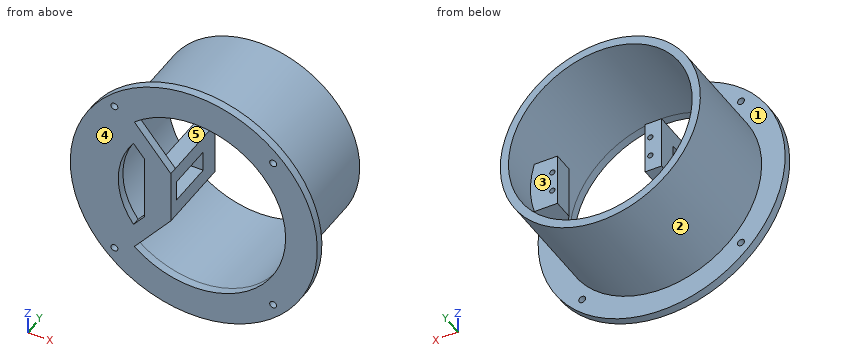
```python
from build123d import *

# Parameters (mm, degrees)
SKETCH1_R           = 60.5
SKETCH1_R_2         = 1.7
BOSS_EXTRUDE1_DEPTH = 4
SKETCH2_R           = 49
SKETCH2_R_2         = 45
BOSS_EXTRUDE2_DEPTH = 53
SKETCH3_W           = 8
SKETCH3_H           = 26
BOSS_EXTRUDE3_DEPTH = 1
SKETCH4_W           = 8
SKETCH4_H           = 8
BOSS_EXTRUDE4_DEPTH = 23
SKETCH5_W           = 8
SKETCH5_H           = 26
BOSS_EXTRUDE5_DEPTH = 10
SKETCH6_R           = 1.3
CUT_EXTRUDE1_DEPTH  = 5
BOSS_EXTRUDE6_START = -10
SKETCH7_R           = 1.3
BOSS_EXTRUDE6_DEPTH = 10
SKETCH12_R          = 1.3
BOSS_EXTRUDE8_DEPTH = 5
RIB4_REACH          = 104.808
SKETCH17_WALL_W     = 226.415050864
SKETCH17_WALL_H     = 26
SKETCH18_R          = 5
CUT_EXTRUDE3_DEPTH  = 21


with BuildPart() as part:
    # Sketch1 → Boss-Extrude1 (new body)
    with BuildSketch(Plane(origin=(0, 0, 0), x_dir=(-1, 0, 0), z_dir=(0, 1, 0))):
        with Locations(Location((0, 0, 0), (0, 0, 90))):
            Circle(SKETCH1_R)
        with Locations(Location((38.890872965, 38.890872965, 0), (0, 0, 90))):
            Circle(SKETCH1_R_2, mode=Mode.SUBTRACT)
        with Locations(Location((38.890872965, -38.890872965, 0), (0, 0, 90))):
            Circle(SKETCH1_R_2, mode=Mode.SUBTRACT)
        with Locations(Location((-38.890872965, -38.890872965, 0), (0, 0, 90))):
            Circle(SKETCH1_R_2, mode=Mode.SUBTRACT)
        with Locations(Location((-38.890872965, 38.890872965, 0), (0, 0, 90))):
            Circle(SKETCH1_R_2, mode=Mode.SUBTRACT)
        with BuildLine():
            Line((11.25, -13), (11.25, 13))
            Line((11.25, 13), (29.125473669, 34.303159964))
            ThreePointArc((29.125473669, 34.303159964), (-45, 0), (29.125473669, -34.303159964))
            Line((29.125473669, -34.303159964), (11.25, -13))
        make_face(mode=Mode.SUBTRACT)
        with BuildLine():
            Line((24.25, -16), (24.25, 16))
            Line((24.25, 16), (29.530226152, 22.292728487))
            ThreePointArc((29.530226152, 22.292728487), (37, 0), (29.530226152, -22.292728487))
            Line((29.530226152, -22.292728487), (24.25, -16))
        make_face(mode=Mode.SUBTRACT)
    extrude(amount=BOSS_EXTRUDE1_DEPTH)

    # Sketch2 → Boss-Extrude2 (add)
    with BuildSketch(Plane(origin=(0, 4, 0), x_dir=(1, 0, 0), z_dir=(0, 1, 0))):
        with Locations(Location((0, 0, 0), (0, 0, 270))):
            Circle(SKETCH2_R)
        with Locations(Location((0, 0, 0), (0, 0, 130.333286411))):
            Circle(SKETCH2_R_2, mode=Mode.SUBTRACT)
    extrude(amount=BOSS_EXTRUDE2_DEPTH)

    # Sketch3 → Boss-Extrude3 (add)
    with BuildSketch(Plane(origin=(0, 4, 0), x_dir=(1, 0, 0), z_dir=(0, 1, 0))):
        with Locations((-15.25, 0)):
            Rectangle(SKETCH3_W, SKETCH3_H)
    extrude(amount=BOSS_EXTRUDE3_DEPTH)

    # Sketch4 → Boss-Extrude4 (add)
    with BuildSketch(Plane(origin=(0, 5, 0), x_dir=(1, 0, 0), z_dir=(0, 1, 0))):
        with Locations((-15.25, 9)):
            Rectangle(SKETCH4_W, SKETCH4_H)
        with Locations((-15.25, -9)):
            Rectangle(SKETCH4_W, SKETCH4_H)
    extrude(amount=BOSS_EXTRUDE4_DEPTH)

    # Sketch5 → Boss-Extrude5 (add)
    with BuildSketch(Plane(origin=(0, 28, 0), x_dir=(1, 0, 0), z_dir=(0, 1, 0))):
        with Locations((-15.25, 0)):
            Rectangle(SKETCH5_W, SKETCH5_H)
    extrude(amount=BOSS_EXTRUDE5_DEPTH)

    # Sketch6 → Cut-Extrude1 (cut)
    with BuildSketch(Plane(origin=(0, 38, 0), x_dir=(1, 0, 0), z_dir=(0, 1, 0))):
        with Locations(Location((-13.75, 5, 0), (0, 0, 270))):
            Circle(SKETCH6_R)
        with Locations(Location((-13.75, -5, 0), (0, 0, 90))):
            Circle(SKETCH6_R)
    extrude(amount=-CUT_EXTRUDE1_DEPTH, mode=Mode.SUBTRACT)

    # Sketch7 → Boss-Extrude6 (add)
    with BuildSketch(Plane(origin=(0, 38, 0), x_dir=(1, 0, 0), z_dir=(0, 1, 0)).offset(BOSS_EXTRUDE6_START)):
        with BuildLine():
            Line((31.75, 13), (31.75, -13))
            Line((31.75, -13), (47.244047244, -13))
            ThreePointArc((47.244047244, -13), (49, 0), (47.244047244, 13))
            Line((47.244047244, 13), (31.75, 13))
        make_face()
        with Locations(Location((34.25, 5, 0), (0, 0, 270))):
            Circle(SKETCH7_R, mode=Mode.SUBTRACT)
        with Locations(Location((34.25, -5, 0), (0, 0, 270))):
            Circle(SKETCH7_R, mode=Mode.SUBTRACT)
    extrude(amount=BOSS_EXTRUDE6_DEPTH)

    # Sketch12 → Boss-Extrude8 (add)
    with BuildSketch(Plane(origin=(0, 28, 0), x_dir=(-1, 0, 0), z_dir=(0, -1, 0))):
        with Locations(Location((-34.25, 5, 0), (0, 0, 270))):
            Circle(SKETCH12_R)
        with Locations(Location((-34.25, -5, 0), (0, 0, 270))):
            Circle(SKETCH12_R)
    extrude(amount=-BOSS_EXTRUDE8_DEPTH)

    # Sketch17 wall → Rib4 (add, up to next)
    with BuildSketch(Plane(origin=(37.415659229, 20.5, 0), x_dir=(0.602764856689, -0.797918872781, 0), z_dir=(-0.797918872781, -0.602764856689, 0)), mode=Mode.PRIVATE) as rib4_sk1:
        Rectangle(SKETCH17_WALL_W, SKETCH17_WALL_H)
    rib4_tool1 = extrude(rib4_sk1.sketch, amount=-RIB4_REACH, mode=Mode.PRIVATE) - part.part
    add(rib4_tool1.solids().sort_by_distance((37.415659229, 20.5, 0))[0])

    # Sketch18 → Cut-Extrude3 (cut)
    with BuildSketch(Plane(origin=(-38.816562471, 0, -1.698375091), x_dir=(0, 1, 0), z_dir=(0.999044171294917, 0, 0.043712055564257474))):
        with Locations((14, 0)):
            Circle(SKETCH18_R)
    extrude(amount=CUT_EXTRUDE3_DEPTH, mode=Mode.SUBTRACT)


solid = part.part
```
The model under review builds one solid part; all positions refer to its coordinate system, in mm. Face numbers are marked on the shaded views. A direction names the side the tool comes from. Give positions to 0.01 mm unless a question says otherwise; leave off trailing zeros. Write each loop counter-clockwise with the first axis right and the second up, starting at its lowest first coordinate (ties: lowest second). Pieces come first, ordered by that corner, then holes. Notation, with made-up numbers: (-16.5, -7.75) - (28.5, -7.75) arc R17 ccw to (28.5, 4.25) - close; hole circle Ø2 at (73, 71.25). An arc over 180 degrees is marked (long way). Answer in a Markdown table with one row per item. Add a question column.
1. Wall thickness on line 1 along Z through (x, y) = (1.5, 27) (3 decimals); line 2 along X through (y, z) = (35.35, 5); line 3 along Z through (x, y) = (-13, 36): over which ranges is each line inside the solid? List them lowest first. Write a range as [from, to].
2. We need section D-D on z = -26. Write out the cut boundary in (x, y), then the cut area to 3 significant figures.
3. Insertion check: P1, Ø9, axis at x = -14, y = 18, coming from the +Z side; P2, Ø2, axis at x = 38.89, z = -38.89, coming from the -Y side (3 decimals); P3, Ø2, axis at x = 34.5, z = 4.5, coming from the +Y side; P4, Ø4, axis at x = -17, y = 14, coming from the -Z side. Each pin has a flat end and moves straight along its axis. Give the tip position at first contact, or say it passes through.
4. Tool access review of the marked faces 4 and 5: name each direction out of +Z, -Z, +X, -X, +Y, -Y from which nothing blocks a thin tool from reaching the whole face with its end or side.
5. Draft analysis for pull direction Z (two halves, no side actions). For the marked faces 1, 2 and 3, state which applies: +Z half, -Z half, draft (parallel to the pull), parting line (faces both ways), or undercut.
6. We need section C-C on y = 21. Write out the cut boundary in (x, z), then the cut area to 3 significant figures.
7. We need section A-A on z = 0. Write out the cut boundary in (x, y).
8. We need section B-B on x = 25.5. Write out the cut boundary in (y, z), then the cut area to 3 significant figures.
Ans:
| question | item | result |
|---|---|---|
| 1 | line 1 | z = [-48.977, -44.975], [44.975, 48.977] |
| 1 | line 2 | x = [-48.74, -44.72], [-19.25, -15.05], [-12.45, -11.25], [31.75, 32.95], [35.55, 48.74] |
| 1 | line 3 | z = [-47.24, -43.08], [-13, -6.06], [-3.94, 3.94], [6.06, 13], [43.08, 47.24] |
| 2 | outline | (-54.63, 0) - (-22.16, 0) - (-22.16, 4) - (-36.73, 4) - (-36.73, 57) - (-41.53, 57) - (-41.53, 4) - (-54.63, 4) - close; (36.73, 0) - (54.63, 0) - (54.63, 4) - (41.53, 4) - (41.53, 57) - (36.73, 57) - close |
| 2 | area | 711 mm^2 |
| 3 | P1 | stops at z = 48.07 |
| 3 | P2 | passes through |
| 3 | P3 | stops at y = 38 |
| 3 | P4 | stops at z = -46.65 |
| 4 | face 4 | +Z, -Z, +X, -X, -Y |
| 4 | face 5 | +Y |
| 5 | face 1 | draft |
| 5 | face 2 | parting line |
| 5 | face 3 | undercut |
| 6 | outline | circle Ø98 at (0, 0); (-19.25, -13) - (-11.25, -13) - (-11.25, -5) - (-19.25, -5) - close; (-19.25, 5) - (-11.25, 5) - (-11.25, 13) - (-19.25, 13) - close; hole (37.04, -13) - (37.04, 13) - (43.08, 13) arc R45 ccw (long way) to (43.08, -13) - close |
| 6 | area | 1,500 mm^2 |
| 7 | outline | (-60.5, 0) - (-37, 0) - (-37, 4) - (-45, 4) - (-45, 57) - (-49, 57) - (-49, 4) - (-60.5, 4) - close; (-24.25, 0) - (-11.25, 0) - (-11.25, 5) - (-19.25, 5) - (-19.25, 4) - (-24.25, 4) - close; (-19.25, 28) - (-11.25, 28) - (-11.25, 38) - (-19.25, 38) - close; (31.75, 28) - (45, 10.46) - (45, 0) - (60.5, 0) - (60.5, 4) - (49, 4) - (49, 57) - (45, 57) - (45, 38) - (31.75, 38) - close |
| 8 | outline | (0, -54.86) - (4, -54.86) - (4, -41.84) - (57, -41.84) - (57, -37.08) - (0, -37.08) - close; (0, 37.08) - (57, 37.08) - (57, 41.84) - (4, 41.84) - (4, 54.86) - (0, 54.86) - close |
| 8 | area | 647 mm^2 |
